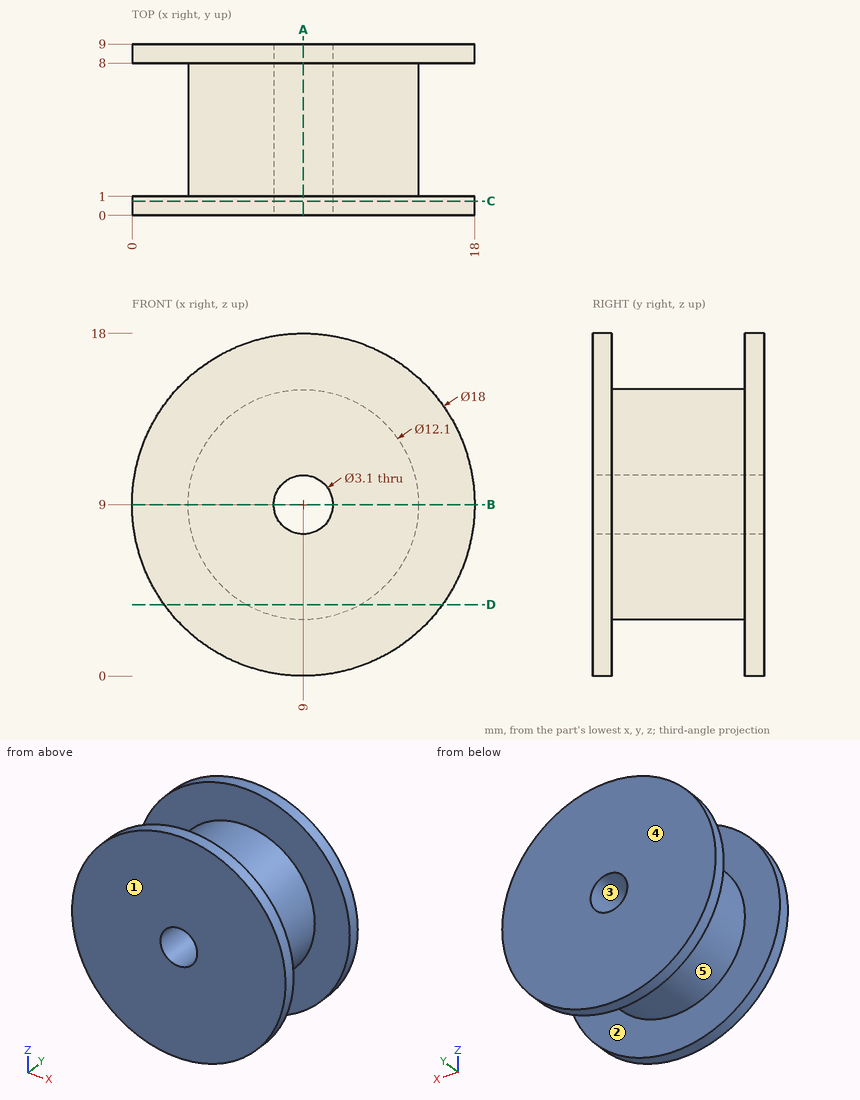
Verification items for this drawing (mm, ordinates from the low corner). A direction names the side the tool comes from. Give positions to 0.01 mm unless a question says otherwise; leave off trailing zeros. Write each loop counter-clockwise with the first axis right and the second up, starting at its lowest first coordinate (ties: lowest second). Pieces come first, ordered by that corner, then holes. Notation, with made-up numbers: (58.5, -15) - (113.5, -15) arc R12 ccw to (113.5, -7) - close; hole circle Ø5 at (77.25, -2). An arc over 180 degrees is marked (long way). Answer as a JSON object with one key per item and string values. Group by question number.
1) Depth check by flat-ended pin: P1, Ø5, axis at x = 4, y = 1.5, coming from the -Z side; P2, Ø1.9, axis at x = 9, z = 9, coming from the -Y side; P3, Ø1, axis at y = 8, z = 6.5, coming from the -X side; P4, Ø5, axis at x = 7, y = 4.5, coming from the -Z side. Enter the tip coordinate at first touch or a pass-through.
2) Sectioned sample at B-B (z = 9). Record the cut outline in (x, y), then the cut area to 3 significant figures.
3) Sectioned sample at C-C (y = 0.75). Record the cut outline in (x, z).
4) Sectioned sample at D-D (z = 3.75). Record the cut outline in (x, y), then the cut area to 3 significant figures.
5) Thickness scan on probe 1 along Y at (x, z) = (3.75, 4); probe 2 along X at (y, z) = (2.5, 9). Record the ranges inside material, lowest first. Write a range as from..to.
6) Release check for a two-part mould opening along Y. For the marked faces 1, 2 and 3 record: pulls with the +Y half, pulls with the -Y half, needs draft (parallel to the pull), parting line crosses it, or undercut.
7) Access from +Z, -Z, +X, -X, +Y, -Y to the whole of each face (thin tool, end or side, straight path). Record for the marked faces 4 and 5.
8) Sectioned sample at A-A (x = 9). Record the cut outline in (y, z).
Geometry results:
{
 "1": {"P1": "stops at z = 0.37", "P2": "passes through", "P3": "stops at x = 0.23", "P4": "stops at z = 2.95"},
 "2": {"outline": "(0, 0) - (7.45, 0) - (7.45, 9) - (0, 9) - (0, 8) - (2.95, 8) - (2.95, 1) - (0, 1) - close; (10.55, 0) - (18, 0) - (18, 1) - (15.05, 1) - (15.05, 8) - (18, 8) - (18, 9) - (10.55, 9) - close", "area": "92.8 mm^2"},
 "3": {"outline": "circle Ø18 at (9, 9); hole circle Ø3.1 at (9, 9)"},
 "4": {"outline": "(1.69, 0) - (16.31, 0) - (16.31, 1) - (12.01, 1) - (12.01, 8) - (16.31, 8) - (16.31, 9) - (1.69, 9) - (1.69, 8) - (5.99, 8) - (5.99, 1) - (1.69, 1) - close", "area": "71.3 mm^2"},
 "5": {"probe 1": "y = 0..1, 8..9", "probe 2": "x = 2.95..7.45, 10.55..15.05"},
 "6": {"face 1": "pulls with the -Y half", "face 2": "undercut", "face 3": "needs draft"},
 "7": {"face 4": "+Z, -Z, +X, -X, +Y", "face 5": "none"},
 "8": {"outline": "(0, 0) - (1, 0) - (1, 2.95) - (8, 2.95) - (8, 0) - (9, 0) - (9, 7.45) - (0, 7.45) - close; (0, 10.55) - (9, 10.55) - (9, 18) - (8, 18) - (8, 15.05) - (1, 15.05) - (1, 18) - (0, 18) - close"}
}
